Autodesk Inventor part; units mm, degrees
ref_plane "YZ Plane" through (0, 0, 0) normal (1, 0, 0) x (0, 1, 0)
ref_plane "XZ Plane" through (0, 0, 0) normal (0, 1, 0) x (-1, 0, 0)
ref_plane "XY Plane" through (0, 0, 0) normal (0, 0, 1) x (1, 0, 0)
sketch "Sketch1" plane through (0, 0, 0) normal (0, 0, 1) x (1, 0, 0)
  line L0 (0, 0) -> (100, 0)
  line L1 (100, 0) -> (100, 20)
  line L2 (0, 0) -> (0, 100)
  line L3 (0, 100) -> (20, 100)
  line L4 (20, 100) -> (20, 20)
  line L5 (20, 20) -> (100, 20)
  dimension "d0" = 100
  dimension "d1" = 20
  dimension "d2" = 100
  dimension "d3" = 20
extrude "Extrusion1" add sketch "Sketch1" along normal mid plane 30
fillet "Fillet1" radius 2 1 edges at (20, 20, 0)
properties part number "CE-10.1.3" material "Stainless Steel"
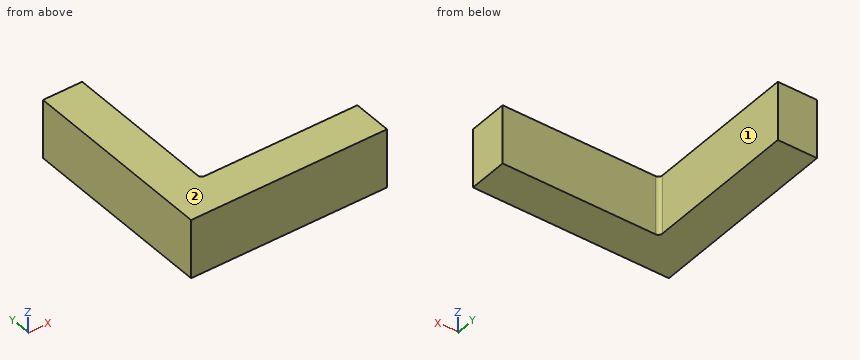
Model file for the job. Use its own axes, mm. Face numbers are marked on the shaded views. A direction names the side the tool comes from. Give positions to 0.01 mm unless a question says otherwise; leave off trailing zeros. Order: outer loops, then holes, each group sorted by start corner. A loop starts at its lowest first (then second) coordinate and runs counter-clockwise, first axis right, second up. Notation, with made-up numbers: M 85,-8 L 133,-8 A15 ccw 133,1 Z; hole C 21,29.5 d7. An arc over 180 degrees is marked long. Put each result on its own line as item: value. Start each with the question number.
(1) Drill centre lines: L1, parallel to Y at x = 59, z = -5.5; L2, parallel to X at y = 21.5, z = 5.25. Where is each one in solid material? Low to high. Write a range as [from, to].
(2) Pin check, flat tips, straight feed: pin 1 Ø4 at (y, z) = (38.5, -2) entering from -X; pin 2 Ø9 at (y, z) = (74.5, 1) entering from +X. Stop position of each tip, or through.
(3) Band-saw the part on B-B on x = 48.5. Give the cut face in (y, z), then the cut area to 3 significant figures.
(4) Tool access for the marked faces 1 and 2: list every direction of +Z, -Z, +X, -X, +Y, -Y with a clear straight run to the whole face (end or side of a thin tool).
(5) Band-saw the part on A-A on z = 9.5. Give the cut face in (x, y).
Results below:
1. L1: y = [0, 20]
1. L2: x = [0, 20.06]
2. pin 1: stops at x = 0
2. pin 2: stops at x = 20
3. outline: M 0,-15 L 20,-15 L 20,15 L 0,15 Z
3. area: 600 mm2
4. face 1: +Z, -Z, +X, +Y
4. face 2: +Z, +X, -X, +Y, -Y
5. outline: M 0,0 L 100,0 L 100,20 L 22,20 A2 cw 20,22 L 20,100 L 0,100 Z
